Study the drawing (mm; zero at the part's minimum x, y, z) and answer. A direction names the side the tool comes from. Coordinates: 2 decimals unless noted, no trailing zeros. Order: outer loops, then holes, each group sorted by start corner. A loop starts at its lowest first (then second) coordinate and runs counter-clockwise, first axis right, second up.
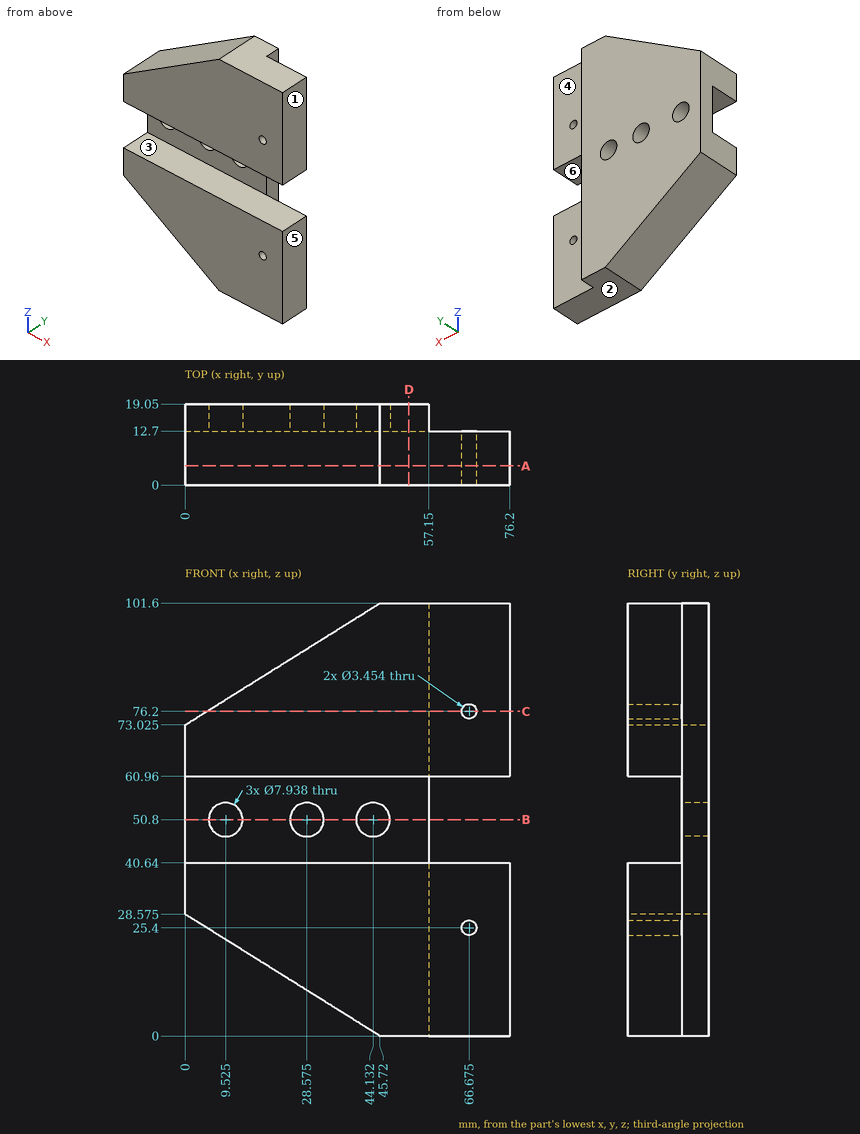
1) A cutting plane is placed at D-D, the plane x = 52.5. Determine the outline of the cut face in (y, z).
A:
outline: (0, 0) - (19.05, 0) - (19.05, 101.6) - (0, 101.6) - (0, 60.96) - (12.7, 60.96) - (12.7, 40.64) - (0, 40.64) - close
2) Which of the six approach directions +Z, -Z, +X, -X, +Y, -Y give full straight-line access (tool end or side, diameter ignored) to the marked faces 4, 5 and 6?
A:
face 4: +Z, -Z, +X, +Y
face 5: +Z, -Z, +X, +Y, -Y
face 6: +X, -X, -Y
3) Flat-ended cylindrical pins translate along their axes: pin 1 Ø10 at (x, y) = (25.5, 5) entering from -Z; pin 2 Ø6 at (y, z) = (2, 91.5) entering from -X; pin 3 Ø5.5 at (x, z) = (65, 80.5) entering from +Y; pin 4 Ø2 at (x, y) = (68, 8) entering from -Z. Find the tip coordinate at first contact, or state that the pin passes through.
A:
pin 1: stops at z = 9.51
pin 2: stops at x = 24.76
pin 3: stops at y = 12.7
pin 4: stops at z = 0
4) A cutting plane is placed at C-C, the plane z = 76.2. Determine the outline of the cut face in (x, y).
A:
outline: (5.08, 0) - (64.95, 0) - (64.95, 12.7) - (57.15, 12.7) - (57.15, 19.05) - (5.08, 19.05) - close; (68.4, 0) - (76.2, 0) - (76.2, 12.7) - (68.4, 12.7) - close
5) A cutting plane is placed at B-B, the plane z = 50.8. Determine the outline of the cut face in (x, y).
A:
outline: (0, 12.7) - (5.56, 12.7) - (5.56, 19.05) - (0, 19.05) - close; (13.49, 12.7) - (24.61, 12.7) - (24.61, 19.05) - (13.49, 19.05) - close; (32.54, 12.7) - (40.16, 12.7) - (40.16, 19.05) - (32.54, 19.05) - close; (48.1, 12.7) - (57.15, 12.7) - (57.15, 19.05) - (48.1, 19.05) - close
6) Determine the mould class of the marked faces 1, 2 and 3 for opening direction Z: pulls with the +Z half, pulls with the -Z half, needs draft (parallel to the pull), parting line crosses it, or undercut.
A:
face 1: needs draft
face 2: pulls with the -Z half
face 3: undercut
7) A cutting plane is placed at A-A, the plane y = 4.5. Determine the outline of the cut face in (x, z) (1 decimal).
A:
outline: (0, 28.6) - (45.7, 0) - (76.2, 0) - (76.2, 40.6) - (0, 40.6) - close; (0, 61) - (76.2, 61) - (76.2, 101.6) - (45.7, 101.6) - (0, 73) - close; hole circle Ø3.5 at (66.7, 25.4); hole circle Ø3.5 at (66.7, 76.2)
8) Straight lines are drawn through the part: line 1 (X direction, y = 16.25, z = 50.8); line 2 (Z direction, x = 61.5, y = 3.5); line 3 (Z direction, x = 30.5, y = 4.75). For each, find the intervals that lie inside material, in ascending order.
A:
line 1: x = 0 to 5.56, 13.49 to 24.61, 32.54 to 40.16, 48.1 to 57.15
line 2: z = 0 to 40.64, 60.96 to 101.6
line 3: z = 9.51 to 40.64, 60.96 to 92.09
